from build123d import *

# Parameters (mm, degrees)
F0_W      = 200
F0_H      = 80
F1_DEPTH  = 10
F2_W      = 42
F2_H      = 22
F3_DEPTH  = 10.001
F5_DEPTH  = 10.001
F6_R      = 3.5
F7_DEPTH  = 10.001
F8_R      = 5
F11_W     = 70
F11_H     = 20
F11_H_2   = 40
F9_W      = 12.4
F9_H      = 11.4
F12_DEPTH = 10.001
F13_R     = 5
F14_W     = 71
F14_H     = 24.5
F15_DEPTH = 10.001


with BuildPart() as f1:
    # F0 (on Top) → F1 (new body)
    with BuildSketch(Plane.XY):
        Rectangle(F0_W, F0_H)
    extrude(amount=F1_DEPTH)

    # F2 (on face) → F3 (cut, through all)
    with BuildSketch(Plane.XY.offset(10)):
        with Locations((-57.7500068545, 10)):
            Rectangle(F2_W, F2_H)
    extrude(amount=-F3_DEPTH, mode=Mode.SUBTRACT)

    # F4 (on face) → F5 (cut, through all)
    with BuildSketch(Plane.XY.offset(10)):
        with BuildLine():
            Line((-81.6500068545, 12.85), (-81.6500068545, 15.1))
            Line((-81.6500068545, 15.1), (-79.4000068545, 15.1))
            ThreePointArc((-79.4000068545, 15.1), (-83.2409971122, 16.6909902577), (-81.6500068545, 12.85))
        make_face()
        with BuildLine():
            Line((-79.4000068545, 15.1), (-81.6500068545, 15.1))
            Line((-81.6500068545, 15.1), (-81.6500068545, 12.85))
            ThreePointArc((-81.6500068545, 12.85), (-80.0590165969, 13.5090097423), (-79.4000068545, 15.1))
        make_face()
        with BuildLine():
            Line((-81.6500068545, 4.9), (-81.6500068545, 7.15))
            ThreePointArc((-81.6500068545, 7.15), (-83.2409971122, 3.3090097423), (-79.4000068545, 4.9))
            Line((-79.4000068545, 4.9), (-81.6500068545, 4.9))
        make_face()
        with BuildLine():
            ThreePointArc((-79.4000068545, 4.9), (-80.0590165969, 6.4909902577), (-81.6500068545, 7.15))
            Line((-81.6500068545, 7.15), (-81.6500068545, 4.9))
            Line((-81.6500068545, 4.9), (-79.4000068545, 4.9))
        make_face()
        with BuildLine():
            Line((-33.8500068545, 15.1), (-36.1000068545, 15.1))
            ThreePointArc((-36.1000068545, 15.1), (-35.4409971122, 13.5090097423), (-33.8500068545, 12.85))
            Line((-33.8500068545, 12.85), (-33.8500068545, 15.1))
        make_face()
        with BuildLine():
            ThreePointArc((-31.6000068545, 15.1), (-33.8500068545, 17.35), (-36.1000068545, 15.1))
            Line((-36.1000068545, 15.1), (-33.8500068545, 15.1))
            Line((-33.8500068545, 15.1), (-33.8500068545, 12.85))
            ThreePointArc((-33.8500068545, 12.85), (-32.2590165969, 13.5090097423), (-31.6000068545, 15.1))
        make_face()
        with BuildLine():
            ThreePointArc((-33.8500068545, 7.15), (-35.4409971122, 6.4909902577), (-36.1000068545, 4.9))
            Line((-36.1000068545, 4.9), (-33.8500068545, 4.9))
            Line((-33.8500068545, 4.9), (-33.8500068545, 7.15))
        make_face()
        with BuildLine():
            Line((-33.8500068545, 4.9), (-36.1000068545, 4.9))
            ThreePointArc((-36.1000068545, 4.9), (-33.8500068545, 2.65), (-31.6000068545, 4.9))
            ThreePointArc((-31.6000068545, 4.9), (-32.2590165969, 6.4909902577), (-33.8500068545, 7.15))
            Line((-33.8500068545, 7.15), (-33.8500068545, 4.9))
        make_face()
    extrude(amount=-F5_DEPTH, mode=Mode.SUBTRACT)

    # F6 (on face) → F7 (cut, through all)
    with BuildSketch(Plane.XY.offset(10)):
        with Locations((-88.3175069503, 30)):
            Circle(F6_R)
        with Locations((12.1812492609, 30)):
            Circle(F6_R)
    extrude(amount=-F7_DEPTH, mode=Mode.SUBTRACT)

    # F8
    f8_edges = [f1.edges().sort_by_distance(p)[0] for p in [
        (-100, 40, 5),
        (-100, -40, 5),
        (100, 40, 5),
        (100, -40, 5),
    ]]
    fillet(f8_edges, radius=F8_R)

    # F11 (on face) + F10 (on face) + F9 (on face) → F12 (cut, through all)
    with BuildSketch(Plane.XY.offset(10)):
        with Locations((65, 30)):
            Rectangle(F11_W, F11_H)
        with Locations((65, -20)):
            Rectangle(F11_W, F11_H_2)
    with BuildSketch(Plane.XY.offset(10)):
        with BuildLine():
            ThreePointArc((93.6749931455, 10), (91.2499931455, 12.425), (88.8249931455, 10))
            Line((88.8249931455, 10), (91.2499931455, 10))
            Line((91.2499931455, 10), (91.2499931455, 7.575))
            ThreePointArc((91.2499931455, 7.575), (92.9647270898, 8.2852660556), (93.6749931455, 10))
        make_face()
        with BuildLine():
            Line((91.2499931455, 10), (88.8249931455, 10))
            ThreePointArc((88.8249931455, 10), (89.5352592011, 8.2852660556), (91.2499931455, 7.575))
            Line((91.2499931455, 7.575), (91.2499931455, 10))
        make_face()
    with BuildSketch(Plane.XY.offset(10)):
        with Locations((6.2, -25.7)):
            Rectangle(F9_W, F9_H)
    extrude(amount=-F12_DEPTH, mode=Mode.SUBTRACT)

    # F13
    f13_edges = [f1.edges().sort_by_distance(p)[0] for p in [
        (30, 40, 5),
        (30, 20, 5),
        (100, 20, 5),
        (30, -40, 5),
        (100, 0, 5),
        (30, 0, 5),
    ]]
    fillet(f13_edges, radius=F13_R)

    # F14 (on face) → F15 (cut, through all)
    with BuildSketch(Plane.XY.offset(10)):
        with Locations((-54.5, -22.25)):
            Rectangle(F14_W, F14_H)
    extrude(amount=-F15_DEPTH, mode=Mode.SUBTRACT)


solid = f1.part
CAD build for the part. Positions are in the model's coordinates, mm. A direction names the side the tool comes from. Coordinates: 2 decimals unless noted, no trailing zeros. Write each loop counter-clockwise with the first axis right and the second up, starting at its lowest first coordinate (ties: lowest second). Pieces come first, ordered by that corner, then holes. Notation, with made-up numbers: M 12,18 L 68,18 A27 cw 68,36 Z; hole C 52.25,-37 d1. An arc over 180 degrees is marked long. Return JSON: item names as keys, results as strings.
Item 1: Drop flat-ended pins along their axis: pin 1 Ø2.5 at (x, y) = (-81.65, 15.1) entering from -Z; pin 2 Ø3 at (y, z) = (-8, 4.5) entering from +X; pin 3 Ø5 at (x, z) = (64.5, 4) entering from -Y; pin 4 Ø3 at (y, z) = (20, 5.5) entering from +X. Give the stop position or say it passes through.
Findings below:
{"pin 1": "passes through", "pin 2": "stops at x = 30", "pin 3": "stops at y = 0", "pin 4": "stops at x = 98.57"}
Item 2: Which spindle directions (+Z, -Z, +X, -X, +Y, -Y) get a long thin tool onto all of the face, cutting with end or side? Do faces 1 (the flat face through (65, 0, 5)), 2 (the flat face through (-58, 21, 5)), 3 (the flat face through (-36, 40, 5)). Say none if no direction does.
Findings below:
{"face 1": "+Z, -Z, +X, -Y", "face 2": "+Z, -Z", "face 3": "+Z, -Z, +X, -X, +Y"}
Item 3: Slice it at A-A, the plane x = -46. Write the cut outline in (y, z).
Findings below:
{"outline": "M -40,0 L -34.5,0 L -34.5,10 L -40,10 Z; M -10,0 L -1,0 L -1,10 L -10,10 Z; M 21,0 L 40,0 L 40,10 L 21,10 Z"}
Item 4: Two-plate mould, pull along Y, no slides. Class faces 4 (the flat face through (0, -26, 5)), 5 (the cylindrical face through (98, 19, 5)), 6 (the cylindrical face through (99, 2, 5)): +Y half, -Y half, draft (parallel to the pull), parting line (faces both ways), or undercut.
Findings below:
{"face 4": "undercut", "face 5": "+Y half", "face 6": "-Y half"}
Item 5: Slice it at D-D, the plane x = 85. Write the cut outline in (y, z), and give its area (3 significant figures).
Findings below:
{"outline": "M 0,0 L 20,0 L 20,10 L 0,10 Z", "area": "200 mm2"}
Item 6: Slice it at B-B, the plane y = 30. Write the cut outline in (x, z), and give its area (3 significant figures).
Findings below:
{"outline": "M -100,0 L -91.82,0 L -91.82,10 L -100,10 Z; M -84.82,0 L 8.68,0 L 8.68,10 L -84.82,10 Z; M 15.68,0 L 30,0 L 30,10 L 15.68,10 Z", "area": "1,160 mm2"}
Item 7: Probe line 1 (X direction, y = -26.5, z = 6.25); line 2 (X direction, y = 15.1, z = 7.5); line 3 (Y direction, x = -70.5, z = 1.5). List the from-to ranges inside material, lowest first. Write a range as from..to.
Findings below:
{"line 1": "x = -100..-90, -19..0, 12.4..30", "line 2": "x = -100..-83.9, -79.4..-78.75, -36.75..-36.1, -31.6..100", "line 3": "y = -40..-34.5, -10..-1, 21..40"}
Item 8: Slice it at C-C, the plane z = 3.75. State how many separate pieces and enclosed holes the cut face has, and give its area (3 significant figures).
Findings below:
{"separate pieces": "1", "enclosed holes": "10", "area": "8,810 mm2"}
